Work out the finished part from the listing and answer in its coordinate system (mm). A direction names the side the tool comes from. Coordinates: 2 decimals unless noted, no trailing zeros. Order: outer loops, then holes, each group sorted by start corner. A loop starts at its lowest first (then second) coordinate and runs counter-clockwise, first axis right, second up. Notation, with made-up numbers: M 65.5,37.25 L 95.5,37.25 A29 cw 95.5,61.25 Z; hole C 4.25,80.25 d10. An arc over 180 degrees is marked long. Use a Markdown table: item, result.
Autodesk Inventor part; units mm, degrees
ref_plane "YZ Plane" through (0, 0, 0) normal (1, 0, 0) x (0, 1, 0)
ref_plane "XZ Plane" through (0, 0, 0) normal (0, 1, 0) x (-1, 0, 0)
ref_plane "XY Plane" through (0, 0, 0) normal (0, 0, 1) x (1, 0, 0)
sketch "Эскиз1" plane through (0, 0, 0) normal (0, 0, 1) x (1, 0, 0)
  circle A0 centre (0, 0) radius 90
  dimension "d0" = 180
extrude "Выдавливание1" add sketch "Эскиз1" along normal blind 8
sketch "Эскиз2" plane through (0, 0, 8) normal (0, 0, 1) x (1, 0, 0)
  point P0 (0, 0)
sketch "Эскиз3" plane through (0, 0, 0) normal (0, 0, -1) x (-1, 0, 0)
  circle A0 centre (0, 0) radius 57.5
  dimension "d3" = 115
sketch "Эскиз4" plane through (0, 0, 8) normal (0, 0, 1) x (1, 0, 0)
  circle A0 centre (0, 0) radius 70
  dimension "d4" = 140
extrude "Выдавливание2" add sketch "Эскиз4" along normal blind 65
hole "Отверстие1" at (0, 0, 0) direction (0, 0, 1) diameter 115 end through all
chamfer "Фаска1" distance 2 angle 45 1 edges at (-70, 0, 73)
chamfer "Фаска2" distance 1 angle 45 1 edges at (0, -57.5, 0)
fillet "Сопряжение1" radius 2 1 edges at (-70, 0, 8)
sketch "Эскиз5" plane through (0, 0, 8) normal (0, 0, 1) x (1, 0, 0)
  circle A0 centre (0, 0) radius 80
  circle A1 centre (0, 0) radius 80
  circle A2 centre (0, 0) radius 80
  circle A3 centre (0, 0) radius 80
  circle A4 centre (0, 0) radius 80
  circle A5 centre (0, 0) radius 80
  point P0 (0, 80)
  point P1 (-69.282, 40)
  point P2 (-69.282, -40)
  point P3 (0, -80)
  point P4 (69.282, -40)
  point P5 (69.282, 40)
  dimension "d21" = 160
  dimension "d24" = 360
hole "Отверстие2" at (69.282, 40, 8) at (69.282, -40, 8) at (0, -80, 8) at (-69.282, -40, 8) at (-69.282, 40, 8) at (0, 80, 8) direction (0, 0, -1) diameter 11 end through all
1. Flat-ended cylindrical pins translate along their axes: P1, Ø2, axis at y = 47, z = 45, coming from the +X side; P2, Ø6, axis at x = -31.5, z = 63.5, coming from the -Y side; P3, Ø2, axis at x = -11, z = 11.5, coming from the -Y side; P4, Ø6.5, axis at x = -69.282, y = -40, coming from the -Z side. Find the tip coordinate at first contact, or state that the pin passes through.
Answers below:
| item | result |
|---|---|
| P1 | x = 52.76 |
| P2 | y = -63.94 |
| P3 | y = -69.28 |
| P4 | through |
2. Find the intervals of material crossed by probe 1 along Y at (x, z) = (0, 3.75); probe 2 along Y at (x, z) = (0, 57); probe 3 along Y at (x, z) = (-19.5, 7), in increasing order.
Answers below:
| item | result |
|---|---|
| probe 1 | -90 to -85.5, -74.5 to -57.5, 57.5 to 74.5, 85.5 to 90 |
| probe 2 | -70 to -57.5, 57.5 to 70 |
| probe 3 | -87.86 to -54.09, 54.09 to 87.86 |
3. For a pull along Y with two mould halves and no side action, classify faces 3 (the face through (-67, 27, 8)), 4 (the face through (-69.524, -34.505, 3.944)), 5 (the face through (64.979, -20.463, 72.875)) as +Y half, -Y half, draft (parallel to the pull), parting line (faces both ways), or undercut.
Answers below:
| item | result |
|---|---|
| face 3 | draft |
| face 4 | undercut |
| face 5 | parting line |
4. For faces 1 (the face through (-55.55, 42.594, 40.073)), 2 (the face through (56.133, -12.465, 37.504)), determine the directions among +Z, -Z, +X, -X, +Y, -Y from which every point of the face is accessible in a straight line to the end or side of a thin tool.
Answers below:
| item | result |
|---|---|
| face 1 | +Z |
| face 2 | +Z, -Z |
5. Section B-B on y = 0 is taken. Determine the outline of the cut face in (x, z), then the cut area to 3 significant figures.
Answers below:
| item | result |
|---|---|
| outline | M -90,0 L -58.5,0 L -57.5,1 L -57.5,73 L -68,73 L -70,71 L -70,10 A2 cw -72,8 L -90,8 Z; M 57.5,1 L 58.5,0 L 90,0 L 90,8 L 72,8 A2 cw 70,10 L 70,71 L 68,73 L 57.5,73 Z |
| area | 2,140 mm² |
6. Section D-D on y = -80 is taken. Determine the outline of the cut face in (x, z).
Answers below:
| item | result |
|---|---|
| outline | M -41.23,0 L -5.5,0 L -5.5,8 L -41.23,8 Z; M 5.5,0 L 41.23,0 L 41.23,8 L 5.5,8 Z |
7. Section A-A on x = 0 is taken. Determine the outline of the cut face in (y, z), then the cut area to 3 significant figures.
Answers below:
| item | result |
|---|---|
| outline | M -90,0 L -85.5,0 L -85.5,8 L -90,8 Z; M -74.5,0 L -58.5,0 L -57.5,1 L -57.5,73 L -68,73 L -70,71 L -70,10 A2 cw -72,8 L -74.5,8 Z; M 57.5,1 L 58.5,0 L 74.5,0 L 74.5,8 L 72,8 A2 cw 70,10 L 70,71 L 68,73 L 57.5,73 Z; M 85.5,0 L 90,0 L 90,8 L 85.5,8 Z |
| area | 1,970 mm² |
8. Section C-C on z = 25.5 is taken. Determine the outline of the cut face in (x, y).
Answers below:
| item | result |
|---|---|
| outline | C 0,0 d140; hole C 0,0 d115 |
